Could you check a few things on this model? Use its own coordinates, in mm. Face numbers are marked on the shaded views. A direction names the side the tool comes from. Round coordinates to 2 decimals unless told otherwise and drop trailing zeros. Write each loop counter-clockwise with the first axis right and the second up, starting at its lowest first coordinate (ties: lowest second). Pieces come first, ordered by that corner, then holes. Notation, with made-up numbers: M -32,48.25 L -5,48.25 A24 cw -5,60.25 Z; hole C -36,84 d2. An arc over 180 degrees is marked long. One line per item, written item: value. Start each with the question number.
(1) I want a section at A-A on x = 3.4. Please give me the cut outline in (y, z).
(2) I'm going to push flat-ended pins straight in: pin 1 Ø1 at (x, z) = (1, 4) entering from +Y; pin 2 Ø1.2 at (y, z) = (6, 5) entering from -X; pin 3 Ø2 at (x, y) = (3, -5) entering from -Z. Where does each tip first touch, or does it pass through?
(3) I want a section at C-C on x = 2.5. Please give me the cut outline in (y, z), and give its area (3 significant figures).
(4) Which directions (+Z, -Z, +X, -X, +Y, -Y) give clear straight access to the entire face, cutting with the end or side of a thin tool? Please do the marked faces 1 and 2.
(5) I want a section at D-D on x = 0.45. Please give me the cut outline in (y, z), and give its area (3 significant figures).
(6) If I drill on L1, parallel to Z at x = 1.5, y = -5.75; L2, parallel to Y at x = 0.95, z = -6; L3, parallel to Z at x = 0.3, y = -1.5, over which ranges is the centre line in solid material (lowest first)?
(7) I want a section at B-B on z = -1.75. Please give me the cut outline in (x, y).
```python
from build123d import *

# Parameters (mm, degrees)
F0_R     = 8
F1_DEPTH = 2
F3_DEPTH = 2
F4_R     = 1


with BuildPart() as f1:
    # F0 (on Right) → F1 (new body)
    with BuildSketch(Plane.YZ):
        Circle(F0_R)
    extrude(amount=F1_DEPTH)

    # F2 (on face) → F3 (join)
    with BuildSketch(Plane.YZ.offset(2)):
        Polygon((8, -4.618802), (8, 4.618802), (0, 9.237604), (-8, 4.618802), (-8, -4.618802), (0, -9.237604), align=None)
    extrude(amount=F3_DEPTH)

    # F4
    f4_edges = [f1.edges().sort_by_distance(p)[0] for p in [
        (3, 0, 9.237604),
        (3, 8, 4.618802),
        (3, 8, -4.618802),
        (3, -8, 4.618802),
        (3, -8, -4.618802),
        (3, 0, -9.237604),
        (4, -4, 6.928203),
        (4, -8, 0),
        (4, -4, -6.928203),
        (4, 4, 6.928203),
        (4, 8, 0),
        (4, 4, -6.928203),
    ]]
    fillet(f4_edges, radius=F4_R)


solid = f1.part
```
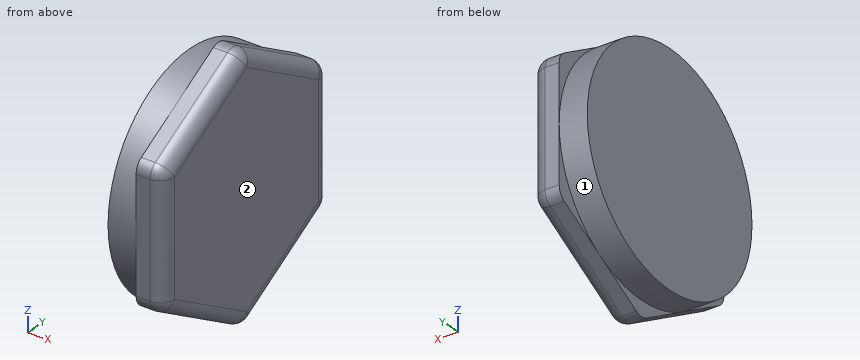
Found:
1. outline: M -7.92,-4.04 A0.92 ccw -7.46,-4.84 L -0.46,-8.88 A0.92 ccw 0.46,-8.88 L 7.46,-4.84 A0.92 ccw 7.92,-4.04 L 7.92,4.04 A0.92 ccw 7.46,4.84 L 0.46,8.88 A0.92 ccw -0.46,8.88 L -7.46,4.84 A0.92 ccw -7.92,4.04 Z
2. pin 1: stops at y = 7.19
2. pin 2: stops at x = 0
2. pin 3: stops at z = -6.93
3. outline: M -8,-4.04 A1 ccw -7.5,-4.91 L -0.5,-8.95 A1 ccw 0.5,-8.95 L 7.5,-4.91 A1 ccw 8,-4.04 L 8,4.04 A1 ccw 7.5,4.91 L 0.5,8.95 A1 ccw -0.5,8.95 L -7.5,4.91 A1 ccw -8,4.04 Z
3. area: 221 mm²
4. face 1: -X
4. face 2: +Z, -Z, +X, +Y, -Y
5. outline: C 0,0 d16
5. area: 201 mm²
6. L1: z = -5.56 to 5.56
6. L2: y = -5.29 to 5.29
6. L3: z = -7.86 to 7.86
7. outline: M 0,-7.81 L 2,-7.81 L 2,-8 L 3,-8 A1 ccw 4,-7 L 4,7 A1 ccw 3,8 L 2,8 L 2,7.81 L 0,7.81 Z
